CAD build for the part. Positions are in the model's coordinates, mm. Face numbers are marked on the shaded views. A direction names the side the tool comes from. Give positions to 0.01 mm unless a question says otherwise; leave off trailing zeros. Write each loop counter-clockwise with the first axis right and the second up, starting at its lowest first coordinate (ties: lowest second). Pieces come first, ordered by that corner, then holes. Notation, with made-up numbers: (42.5, -25.75) - (85.5, -25.75) arc R14 ccw to (85.5, -19.75) - close; hole circle Ø3 at (-7.75, 89). An arc over 180 degrees is marked (long way). Answer as a JSON object with one key per item and string values.
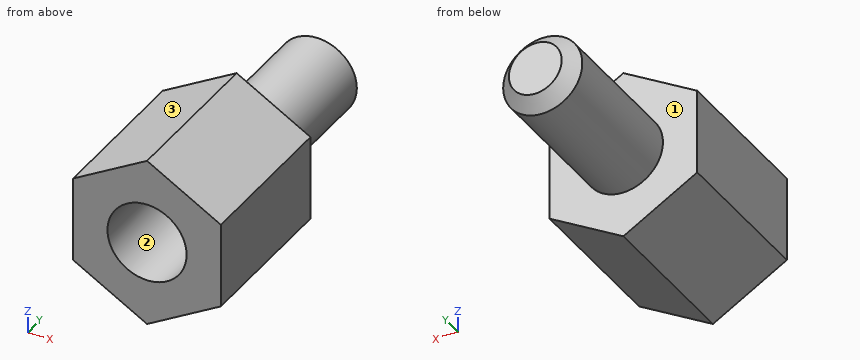
from build123d import *

# Parameters (mm, degrees)
BOSS_EXTRUDE1_DEPTH = 6
SKETCH2_R           = 1.5
BOSS_EXTRUDE2_DEPTH = 5.9
SKETCH3_R           = 1.5
CUT_EXTRUDE1_DEPTH  = 4
CHAMFER1_SIZE       = 0.5


with BuildPart() as part:
    # Sketch1 → Boss-Extrude1 (new body)
    with BuildSketch(Plane(origin=(0, 0, 0), x_dir=(1, 0, 0), z_dir=(0, 1, 0))):
        Polygon((0, -3.233161507), (2.8, -1.616580754), (2.8, 1.616580754), (0, 3.233161507), (-2.8, 1.616580754), (-2.8, -1.616580754), align=None)
    extrude(amount=BOSS_EXTRUDE1_DEPTH)

    # Sketch2 → Boss-Extrude2 (add)
    with BuildSketch(Plane(origin=(0, 6, 0), x_dir=(1, 0, 0), z_dir=(0, 1, 0))):
        Circle(SKETCH2_R)
    extrude(amount=BOSS_EXTRUDE2_DEPTH)

    # Sketch3 → Cut-Extrude1 (cut)
    with BuildSketch(Plane.XZ):
        Circle(SKETCH3_R)
    extrude(amount=-CUT_EXTRUDE1_DEPTH, mode=Mode.SUBTRACT)

    # Chamfer1
    chamfer1_edges = [part.edges().sort_by_distance(p)[0] for p in [
        (-1.5, 11.9, 0),
    ]]
    chamfer(chamfer1_edges, length=CHAMFER1_SIZE)


solid = part.part
(1) Saw through at C-C, the plane y = 5. Give the cut face in (x, z), and give its area (3 significant figures).
Answer key:
{"outline": "(-2.8, -1.62) - (0, -3.23) - (2.8, -1.62) - (2.8, 1.62) - (0, 3.23) - (-2.8, 1.62) - close", "area": "27.2 mm²"}
(2) Probe L1, parallel to Y at x = -0.75, z = 1.75; L2, parallel to Z at x = 0, y = 9.25; L3, parallel to Y at x = -0.8, z = 1. List the from-to ranges inside material, lowest first. Write a range as [from, to].
Answer key:
{"L1": "y = [0, 6]", "L2": "z = [-1.5, 1.5]", "L3": "y = [4, 11.62]"}
(3) 3-axis set-ups, long thin cutter, end or side, ignore diameter. For the marked faces 1, 2 and 3: which of +Z, -Z, +X, -X, +Y, -Y reach the whole face in a straight line?
Answer key:
{"face 1": "+Y", "face 2": "-Y", "face 3": "+Z, -X, +Y, -Y"}
(4) Saw through at A-A, the plane y = 3. Give the cut face in (x, z), and give its area (3 significant figures).
Answer key:
{"outline": "(-2.8, -1.62) - (0, -3.23) - (2.8, -1.62) - (2.8, 1.62) - (0, 3.23) - (-2.8, 1.62) - close; hole circle Ø3 at (0, 0)", "area": "20.1 mm²"}
(5) Flat gauge pins, fed straight in: P1, Ø1, axis at x = -1.5, y = 10, coming from the -Z side; P2, Ø1.5, axis at x = 0.5, z = -0.5, coming from the -Y side; P3, Ø3, axis at x = -2, y = 3, coming from the -Z side. Where does each tip first touch, or does it go through?
Answer key:
{"P1": "stops at z = -1.12", "P2": "stops at y = 4", "P3": "stops at z = -2.94"}
(6) Saw through at D-D, the plane x = 1.8. Give the cut face in (y, z).
Answer key:
{"outline": "(0, -2.19) - (6, -2.19) - (6, 2.19) - (0, 2.19) - close"}
(7) Saw through at B-B, the plane z = 0. Give the cut face in (x, y).
Answer key:
{"outline": "(-2.8, 0) - (-1.5, 0) - (-1.5, 4) - (1.5, 4) - (1.5, 0) - (2.8, 0) - (2.8, 6) - (1.5, 6) - (1.5, 11.4) - (1, 11.9) - (-1, 11.9) - (-1.5, 11.4) - (-1.5, 6) - (-2.8, 6) - close"}
